CAD build for the part. Positions are in the model's coordinates, mm. Face numbers are marked on the shaded views. Round coordinates to 2 decimals unless told otherwise and drop trailing zeros. Write each loop counter-clockwise with the first axis right and the second up, starting at its lowest first coordinate (ties: lowest second). Pieces come first, ordered by that corner, then holes. Notation, with made-up numbers: (-39, -8.5) -> (-20, -8.5) arc R28 cw to (-20, 26.5) -> close; hole circle Ø9 at (70.25, -23.75). An arc over 180 degrees is marked (long way). Put each result on its own line as item: value. Start each with the question number.
1. Saw through at A-A on x = 0. List the corners of the cut face in (y, z), and give its area (3 significant figures).
2. Pull direction Y, two halves, no side cores. Call the marked faces 1, 2, 3 and 4: pulls with the +Y half, pulls with the -Y half, needs draft (parallel to the pull), parting line crosses it, or undercut.
3. Saw through at B-B on z = -0.3. List the corners of the cut face in (x, y).
4. Flat gauge pin, fed straight in: P1, Ø1, axis at x = 0, y = -1, coming from the +Z side. Where does the tip first touch, or does it go through?
5. Drill centre lines: line 1 (Y direction, x = 0, z = 0.2); line 2 (Y direction, x = -0.5, z = 1.15); line 3 (X direction, y = -1.25, z = -0.8). Where is each one in solid material? Low to high. Write a range as from..to.
6. Saw through at C-C on z = 1.05. List the corners of the cut face in (x, y).
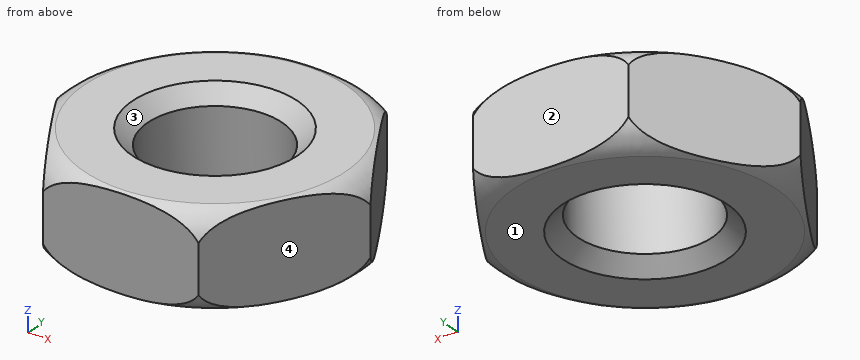
Autodesk Inventor part; units mm, degrees
ref_plane "YZ Plane" through (0, 0, 0) normal (1, 0, 0) x (0, 1, 0)
ref_plane "XZ Plane" through (0, 0, 0) normal (0, 1, 0) x (-1, 0, 0)
ref_plane "XY Plane" through (0, 0, 0) normal (0, 0, 1) x (1, 0, 0)
sketch "Sketch1" plane through (0, 0, 0) normal (0, 0, 1) x (1, 0, 0)
  line L0 (-4.0776, 0) -> (11.9806, 0)
  line L1 (0, 5.675) -> (0, -5.0865)
  line L2 (-3.6188, 3.5) -> (4.159, 3.5)
  line L3 (-3.3522, -3.5) -> (4.4256, -3.5)
  line L4 (-1.2217, -4.8839) -> (-5.1106, 1.8518)
  line L5 (4.7072, -1.1531) -> (0.8183, 5.5827)
  line L6 (4.8405, 1.3839) -> (0.9516, -5.3518)
  line L7 (-1.355, 4.6531) -> (-5.2439, -2.0827)
  circle A0 centre (0, 0) radius 1.75
  point P0 (4.0415, 0)
  point P1 (2.0207, 3.5)
  point P2 (-2.0207, 3.5)
  point P3 (-4.0415, 0)
  point P4 (-2.0207, -3.5)
  point P5 (2.0207, -3.5)
  dimension "d0" = 7
  dimension "d3" = 360
  dimension "d5" = 3.5
extrude "Extrusion1" add sketch "Sketch1" along normal mid plane 2.5 contours L7 L2 L1 A0 L0 | L0 A0 L1 L3 L4 | L1 L2 L5 L0 A0 | A0 L0 L6 L3 L1
sketch "Sketch2" plane through (0, 0, 0) normal (0, 1, 0) x (-1, 0, 0)
  circle A0 centre (3.1105, -0.3099) radius 0.984
  line L0 (0, -2.0822) -> (0, 3.6497)
  line L1 (2.0207, -1.25) -> (4.0415, -1.25)
  line L2 (3.4011, -1.25) -> (4.0415, -1.25)
  line L3 (4.0415, -1.25) -> (4.0415, 0.0088)
  point P0 (0, 0)
  point P1 (4.0415, -0.6286)
  point P2 (2.8198, -1.25)
  dimension "d11" = 1.968
  dimension "d12" = 0.9401
  dimension "d13" = 0.931
revolve "Revolution1" cut sketch "Sketch2" angle 360 about axis through (0, 0, -2.0822) along (0, 0, 1) picked at (3.9263, -1.0343) contours L3 L1 A0 | L1 A0
mirror "Mirror1" about plane through (0, 0, 0) normal (0, 0, 1) of "Revolution1"
thread "Thread1"
chamfer "Chamfer1" distance 0.4 angle 45 1 edges at (-1.75, 0, 1.25)
chamfer "Chamfer2" distance 0.4 angle 45 1 edges at (-1.75, 0, -1.25)
properties part number "somun"
Return value:
1. outline: (-3.5, -1.21) arc R0.98 ccw to (-3.4, -1.25) -> (-2.15, -1.25) -> (-1.75, -0.85) -> (-1.75, 0.85) -> (-2.15, 1.25) -> (-3.4, 1.25) arc R0.98 ccw to (-3.5, 1.21) -> close; (1.75, -0.85) -> (2.15, -1.25) -> (3.4, -1.25) arc R0.98 ccw to (3.5, -1.21) -> (3.5, 1.21) arc R0.98 ccw to (3.4, 1.25) -> (2.15, 1.25) -> (1.75, 0.85) -> close
1. area: 8.42 mm^2
2. face 1: needs draft
2. face 2: pulls with the +Y half
2. face 3: undercut
2. face 4: pulls with the -Y half
3. outline: (-4.04, 0) -> (-2.02, -3.5) -> (2.02, -3.5) -> (4.04, 0) -> (2.02, 3.5) -> (-2.02, 3.5) -> close; hole circle Ø3.5 at (0, 0)
4. P1: passes through
5. line 1: y = -3.5..-1.75, 1.75..3.5
5. line 2: y = -3.5..-1.99, 1.99..3.5
5. line 3: x = -3.32..-1.22, 1.22..3.32
6. outline: (-3.72, -0.56) -> (-2.35, -2.94) arc R3.76 ccw to (-1.37, -3.5) -> (1.37, -3.5) arc R3.76 ccw to (2.35, -2.94) -> (3.72, -0.56) arc R3.76 ccw to (3.72, 0.56) -> (2.35, 2.94) arc R3.76 ccw to (1.37, 3.5) -> (-1.37, 3.5) arc R3.76 ccw to (-2.35, 2.94) -> (-3.72, 0.56) arc R3.76 ccw to start; hole circle Ø3.9 at (0, 0)
